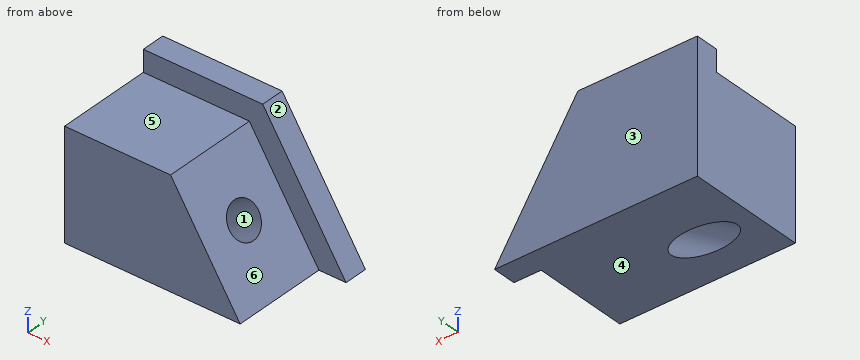
from build123d import *

# Parameters (mm, degrees)
F1_DEPTH = 61.722
F2_DEPTH = 12.192
F3_R     = 9.1987347471
F4_DEPTH = 76.4727140636


with BuildPart() as f1:
    # F0 (on Front) → F1 (new body)
    with BuildSketch(Plane.XZ):
        Polygon((-21.5064492077, 56.3980266452), (-76.2501358986, 56.3980266452), (-76.2501358986, 0), (-21.5064492077, 0), (-14.5882889628, 0), (14.417463594, 0), align=None)
    extrude(amount=F1_DEPTH)

    # F0 (on Front) → F2 (join)
    with BuildSketch(Plane.XZ):
        Polygon((-14.5882889628, 67.5272345543), (-76.2501358986, 67.5272345543), (-76.2501358986, 56.3980266452), (-21.5064492077, 56.3980266452), (14.417463594, 0), (28.4246075898, 0), align=None)
        Polygon((-21.5064492077, 56.3980266452), (-76.2501358986, 56.3980266452), (-76.2501358986, 0), (-21.5064492077, 0), (-14.5882889628, 0), (14.417463594, 0), align=None)
    extrude(amount=F2_DEPTH)

    # F3 (on face) → F4 (cut, through all)
    with BuildSketch(Plane(origin=(10.2561951973, 0, 6.5328998878), x_dir=(0, 1, 0), z_dir=(0.8434293451, 0, 0.5372401137))):
        with Locations((-36.8216447532, 26.6688428819)):
            Circle(F3_R)
    extrude(amount=-F4_DEPTH, mode=Mode.SUBTRACT)


solid = f1.part
The listing builds one solid part. Answer for the finished solid, in the listing's coordinates (mm). Face numbers are marked on the shaded views. A direction names the side the tool comes from. Give positions to 0.01 mm unless a question says otherwise; leave off trailing zeros. Write each loop counter-clockwise with the first axis right and the second up, starting at its lowest first coordinate (ties: lowest second). Pieces come first, ordered by that corner, then holes. Notation, with made-up numbers: (45.25, -21) - (100.25, -21) arc R28 cw to (100.25, -3) - close; hole circle Ø9 at (32.25, 79). An arc over 180 degrees is marked (long way). One line per question, with ' | ' between items. Start each with the question number.
1. Determine the mould class of the marked faces 1, 2 and 3 for opening direction Y: +Y half, -Y half, draft (parallel to the pull), parting line (faces both ways), or undercut.
2. Section D-D, the plane z = 46.5 is taken. Determine the outline of the cut face in (x, y).
3. Section B-B, the plane y = -6 is taken. Determine the outline of the cut face in (x, z).
4. Section A-A, the plane y = -36.5 is taken. Determine the outline of the cut face in (x, z).
5. Given P1, Ø8, axis at x = -24.5, y = -36, coming from the +Z side; P2, Ø4, axis at y = -24.5, z = 14.5, coming from the +X side; P3, Ø10, axis at x = -7, z = 58, coming from the -Y side, each flat-ended and moving along its own axis, determine where each tip first touches the part or whether it passes through.
6. For the marked faces 4, 5 and 6, determine the directions among +Z, -Z, +X, -X, +Y, -Y from which every point of the face is accessible in a straight line to the end or side of a thin tool.
7. Straight lines are drawn through the part: line 1 (Z direction, x = -54, y = -22); line 2 (Y direction, x = -38, z = 14); line 3 (Y direction, x = 5, z = 36.5). For each, find the intervals that lie inside material, in ascending order.
8. Section C-C, the plane x = 11 is taken. Determine the outline of the cut face in (y, z), then the cut area to 3 significant figures.
Result:
1) face 1: undercut | face 2: draft | face 3: +Y half
2) outline: (-76.25, -61.72) - (-15.2, -61.72) - (-15.2, -12.19) - (-1.19, -12.19) - (-1.19, 0) - (-76.25, 0) - close
3) outline: (-76.25, 0) - (28.42, 0) - (-14.59, 67.53) - (-76.25, 67.53) - close
4) outline: (-76.25, 0) - (-66.75, 0) - (-9.01, 36.78) - (-21.51, 56.4) - (-76.25, 56.4) - close; (-32.53, 0) - (14.42, 0) - (0.87, 21.27) - close
5) P1: stops at z = 56.4 | P2: stops at x = 6.46 | P3: stops at y = -12.19
6) face 4: -Z, +X, -X, +Y, -Y | face 5: +Z, +X, -X, -Y | face 6: +Z, +X, -Y
7) line 1: z = 0 to 56.4 | line 2: y = -61.72 to -44.15, -29.49 to 0 | line 3: y = -12.19 to 0
8) outline: (-61.72, 0) - (0, 0) - (0, 27.36) - (-12.19, 27.36) - (-12.19, 5.37) - (-61.72, 5.37) - close | area: 599 mm2
